```python
from build123d import *

# Parameters (mm, degrees)
F1_DEPTH = 3.175
F2_R     = 20.6375
F2_R_2   = 1.7272
F2_R_3   = 2.15265
F3_DEPTH = 3.175
F4_R     = 2.15265
F5_DEPTH = 3.175


with BuildPart() as f1:
    # F0 (on Top) → F1 (new body)
    with BuildSketch(Plane.XY):
        Polygon((279.4, -920.674486), (279.4, 0), (260.683749, 69.85), (209.55, 120.983749), (139.7, 139.7), (69.85, 120.983749), (18.716251, 69.85), (0, 0), (0, -920.674486), (18.716251, -990.524486), (69.85, -1041.658235), (139.7, -1060.374486), (209.55, -1041.658235), (260.683749, -990.524486), align=None)
    extrude(amount=F1_DEPTH)

    # F2 (on face) → F3 (cut, through all)
    with BuildSketch(Plane.XY.offset(3.175)):
        with Locations((139.7, 69.815902)):
            Circle(F2_R)
        with Locations((229.093993, -31.136842)):
            Circle(F2_R_2)
        with Locations((229.093993, -157.74139)):
            Circle(F2_R_2)
        with Locations((110.33125, 40.447152)):
            Circle(F2_R_2)
        with Locations((169.06875, 40.447152)):
            Circle(F2_R_2)
        with Locations((169.06875, 99.184652)):
            Circle(F2_R_2)
        with Locations((110.33125, 99.184652)):
            Circle(F2_R_2)
        with Locations((50.306007, -157.74139)):
            Circle(F2_R_2)
        with Locations((50.306007, -31.136842)):
            Circle(F2_R_2)
        with Locations((248.34149, -235.726616)):
            Circle(F2_R_2)
        with Locations((31.05851, -235.726616)):
            Circle(F2_R_2)
        with Locations((150.01875, -286.526616)):
            Circle(F2_R_3)
        with Locations((129.38125, -286.526616)):
            Circle(F2_R_3)
        with Locations((129.38125, -253.189116)):
            Circle(F2_R_3)
        with Locations((150.01875, -253.189116)):
            Circle(F2_R_3)
        with Locations((129.38125, -923.681501)):
            Circle(F2_R_3)
        with Locations((150.01875, -923.681501)):
            Circle(F2_R_3)
        with Locations((150.01875, -957.019001)):
            Circle(F2_R_3)
        with Locations((129.38125, -957.019001)):
            Circle(F2_R_3)
        with Locations((139.7, -966.544001)):
            Circle(F2_R_2)
        with Locations((139.7, -1030.044001)):
            Circle(F2_R_2)
    extrude(amount=-F3_DEPTH, mode=Mode.SUBTRACT)

    # F4 (on face) → F5 (cut, through all)
    with BuildSketch(Plane.XY.offset(3.175)):
        with Locations((109.951253, 29.748759)):
            Circle(F4_R)
        with Locations((169.448747, 29.748759)):
            Circle(F4_R)
    extrude(amount=-F5_DEPTH, mode=Mode.SUBTRACT)


solid = f1.part
```
Check sheet for the modelled part. Datum: model origin and axes. Units: mm. Give positions to 0.01 mm unless a question says otherwise; leave off trailing zeros. Order: outer loops, then holes, each group sorted by start corner. A loop starts at its lowest first (then second) coordinate and runs counter-clockwise, first axis right, second up. Notation, with made-up numbers: M -14,80.5 L 35,80.5 A34 ccw 35,118.5 Z; hole C -16,87.5 d1. An arc over 180 degrees is marked long. Answer in a Markdown table with one row per item. Add a question column.
Q1. Thickness scan on L1, parallel to X at y = -286.5, z = 1.7; L2, parallel to Y at x = 139.7, z = 1.45; L3, parallel to Y at x = 158.5, z = 0.7. Record the ranges inside material, lowest first.
Q2. Release check for a two-part mould opening along X. For faces 1 (the flat face through (43.925, -1015.733, 1.565)), 2 (the cylindrical face through (135.23, 49.67, 1.61)), 3 (the flat face through (175.11, 130.21, 1.57)), 4 (the flat face through (138, -452, 3.175)) record: released by +X, released by -X, zero draft, split by the parting line, or undercut.
Q3. Sectioned sample at A-A, the plane z = 1.6. Count the separate pieces of the cut face and the enclosed holes in it, and give its area (3 significant figures).
Q4. Gauge pin test, flat ends, axial feed: pin 1 Ø3 at (x, y) = (229.09, -31.14) entering from +Z; pin 2 Ø1.5 at (x, z) = (181.5, 2) entering from +Y. Record the tip position at first contact, or that the pin passes through.
Q5. Sectioned sample at B-B, the plane x = 191. Record the boundary of the cut face in (y, z) (3 decimals), and give its area (3 significant figures).
Verdict:
| question | item | result |
|---|---|---|
| 1 | L1 | 0 to 127.23, 131.53 to 147.87, 152.17 to 279.4 |
| 1 | L2 | -1060.37 to -1031.77, -1028.32 to -968.27, -964.82 to 49.18, 90.45 to 139.7 |
| 1 | L3 | -1055.34 to 61.3, 78.33 to 134.66 |
| 2 | face 1 | released by -X |
| 2 | face 2 | undercut |
| 2 | face 3 | released by +X |
| 2 | face 4 | zero draft |
| 3 | separate pieces | 1 |
| 3 | enclosed holes | 23 |
| 3 | area | 314,000 mm² |
| 4 | pin 1 | through |
| 4 | pin 2 | y = 128.7 |
| 5 | outline | M -1046.629,0 L 125.954,0 L 125.954,3.175 L -1046.629,3.175 Z |
| 5 | area | 3,720 mm² |
